from build123d import *

# Parameters (mm, degrees)
EXTRUDE1_DEPTH = 88
FILLET1_R      = 1
SKETCH4_R      = 8.45
EXTRUDE2_DEPTH = 0.7
EXTRUDE3_DEPTH = 2.5
SKETCH6_R      = 4.75
EXTRUDE4_DEPTH = 84.8
CHAMFER1_SIZE  = 1
CHAMFER2_SIZE  = 0.5
SKETCH7_R      = 5.75
EXTRUDE5_DEPTH = 0.1
EXTRUDE6_DEPTH = 9
FILLET2_R      = 0.5


with BuildPart() as part:
    # Sketch2 → Extrude1 (new, symmetric)
    with BuildSketch(Plane.XY):
        with BuildLine():
            ThreePointArc((-10.291176471, -1.814989491), (10.45, 0), (-10.291176471, 1.814989491))
            ThreePointArc((-10.291176471, 1.814989491), (-23.95, 0), (-10.291176471, -1.814989491))
        make_face()
    extrude(amount=EXTRUDE1_DEPTH, both=True)

    # Fillet1
    fillet1_edges = [part.edges().sort_by_distance(p)[0] for p in [
        (-10.291176471, 1.814989491, 0),
        (-10.291176471, -1.814989491, 0),
    ]]
    fillet(fillet1_edges, radius=FILLET1_R)

    # Sketch3 → Revolve1 (revolve)
    with BuildSketch(Plane(origin=(0, 0, 0), x_dir=(1, 0, 0), z_dir=(0, 1, 0))):
        Polygon((-20, -88), (-20, -88.8), (-24.05, -88.8), (-24.05, -90.8), (-25.05, -90.8), (-25.05, -97.4), (-19.45, -97.4), (-19.45, -97.1), (-17, -97.1), (-17, -88), align=None)
    revolve(axis=Axis((-17, 0, -88.93192935), (0, 0, 1)))

    # Sketch4 → Extrude2 (cut)
    with BuildSketch(Plane.XY.offset(88)):
        Circle(SKETCH4_R)
    extrude2 = extrude(amount=-EXTRUDE2_DEPTH, mode=Mode.SUBTRACT)

    # Sketch5 → Extrude3 (cut)
    with BuildSketch(Plane.XY.offset(87.3)):
        with BuildLine():
            Line((-6.439880123, 5.470872325), (-4.008084609, 2.549069981))
            ThreePointArc((-4.008084609, 2.549069981), (-3.650918419, -3.038633689), (1.779102837, -4.404235813))
            Line((1.779102837, -4.404235813), (4.210898352, -7.326038157))
            ThreePointArc((4.210898352, -7.326038157), (5.405569405, -6.494791714), (6.439880123, -5.470872325))
            Line((6.439880123, -5.470872325), (4.008084609, -2.549069981))
            ThreePointArc((4.008084609, -2.549069981), (3.650918419, 3.038633689), (-1.779102837, 4.404235813))
            Line((-1.779102837, 4.404235813), (-4.210898352, 7.326038157))
            ThreePointArc((-4.210898352, 7.326038157), (-5.405569405, 6.494791714), (-6.439880123, 5.470872325))
        make_face()
    extrude3 = extrude(amount=-EXTRUDE3_DEPTH, mode=Mode.SUBTRACT)

    # Sketch6 → Extrude4 (cut)
    with BuildSketch(Plane.XY.offset(84.8)):
        Circle(SKETCH6_R)
    extrude4 = extrude(amount=-EXTRUDE4_DEPTH, mode=Mode.SUBTRACT)

    # Mirror1: Extrude2, Extrude3, Extrude4 across plane
    add(extrude2.mirror(Plane.XY), mode=Mode.SUBTRACT)
    add(extrude3.mirror(Plane.XY), mode=Mode.SUBTRACT)
    add(extrude4.mirror(Plane.XY), mode=Mode.SUBTRACT)

    # Chamfer1
    chamfer1_edges = [part.edges().sort_by_distance(p)[0] for p in [
        (-9.95, 0, 88.8),
        (-8.95, 0, 90.8),
    ]]
    chamfer(chamfer1_edges, length=CHAMFER1_SIZE - 0.0001)  # a hair under: the kernel refuses the full size

    # Chamfer2
    chamfer2_edges = [part.edges().sort_by_distance(p)[0] for p in [
        (-8.95, 0, 97.4),
    ]]
    chamfer(chamfer2_edges, length=CHAMFER2_SIZE)

    # Sketch7 → Extrude5 (cut)
    with BuildSketch(Plane(origin=(0, 0, -88), x_dir=(-1, 0, 0), z_dir=(0, 0, -1))):
        with Locations((17, 0)):
            Circle(SKETCH7_R)
    extrude(amount=-EXTRUDE5_DEPTH, mode=Mode.SUBTRACT)

    # Sketch8 → Extrude6 (cut)
    with BuildSketch(Plane(origin=(0, 0, -87.9), x_dir=(-1, 0, 0), z_dir=(0, 0, -1))):
        Polygon((19.383629921, 2.513624554), (16.014952241, 3.321096342), (13.63132232, 0.807471788), (14.616370079, -2.513624554), (17.985047759, -3.321096342), (20.36867768, -0.807471788), align=None)
    extrude(amount=-EXTRUDE6_DEPTH, mode=Mode.SUBTRACT)

    # Fillet2
    fillet2_edges = [part.edges().sort_by_distance(p)[0] for p in [
        (-23.95, 0, -88),
        (-23.95, 0, 88),
        (-10.396212718, -3.578308658, -88),
        (-10.396212718, -3.578308658, 88),
        (-10.396212718, 3.578308658, -88),
        (-10.396212718, 3.578308658, 88),
        (10.45, 0, -88),
        (10.45, 0, 88),
    ]]
    fillet(fillet2_edges, radius=FILLET2_R)


solid = part.part
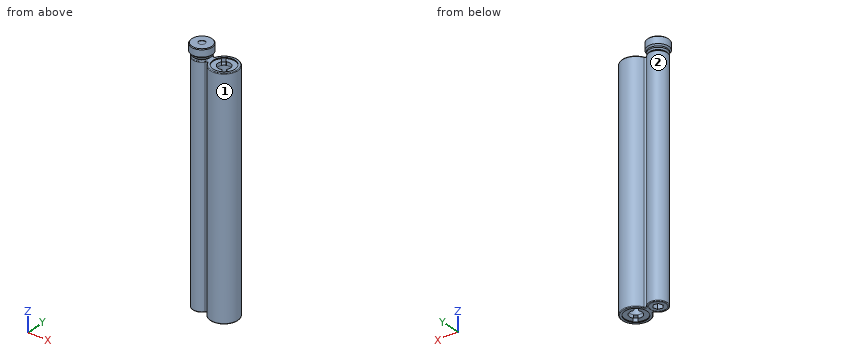
Input: part model. Units: mm. Frame: model coordinates. Face numbers are marked on the shaded views. A direction names the side the tool comes from. Round coordinates to 2 decimals unless told otherwise and drop trailing zeros. Answer as a JSON object with one key per item and string values. Group by question number.
1) Ray query, L1, parallel to Y at x = 0, z = 65; L2, parallel to X at y = 0, z = -87.55; L3, parallel to X at y = 0, z = 46. Return the intervals inside material, ascending.
2) Reachability of the marked faces 1 and 2 from +Z, -Z, +X, -X, +Y, -Y: full face, straight path, thin tool, end or side. Return the list, or none.
3) Pin query (flat end, axial travel): pin 1 (3.5 mm diameter, centred on x = -18.5, y = -0.5, fed in from -Z); pin 2 (2 mm diameter, centred on y = -4, z = -56, fed in from +X); pin 3 (7.5 mm diameter, centred on x = -18.5, y = 1.5, fed in from -Z); pin 4 (8 mm diameter, centred on y = 5, z = -6.5, fed in from -X). Return the tip coordinate at first contact, or that it passes through.
Reply:
{
 "1": {"L1": "y = -10.45 to -4.75, 4.75 to 10.45", "L2": "x = -23.95 to -20.13, -13.87 to -8.45, 8.45 to 10.45", "L3": "x = -23.95 to -4.75, 4.75 to 10.45"},
 "2": {"face 1": "+Z, -Z", "face 2": "-Z"},
 "3": {"pin 1": "stops at z = -87.9", "pin 2": "stops at x = 10.01", "pin 3": "stops at z = -88", "pin 4": "stops at x = -23.88"}
}
